Design review of the part built by this model. Coordinates are the model's own, in mm. Face numbers are marked on the shaded views. A direction names the side the tool comes from. Coordinates: 2 decimals unless noted, no trailing zeros. Loops run counter-clockwise (first coordinate to the right, second up) from the corner with the lowest first, then second, coordinate; pieces in that order, holes last. Notation, with made-up numbers: (67, -22.75) - (126, -22.75) arc R11 ccw to (126, -17.75) - close; hole circle Ø8 at (75.25, 35). An arc over 180 degrees is marked (long way). Answer in a Markdown table with one row per item. Add a question column.
(1) Clearance check with flat-ended pins moving along their axes: pin 1 (5.5 mm diameter, centred on x = 31, y = 24.5, fed in from +Z); pin 2 (1.5 mm diameter, centred on y = 5.5, z = 38, fed in from +X); pin 3 (9.5 mm diameter, centred on x = 36, y = 29, fed in from -Z). State where each tip first meets the part, or that it passes through.
(2) To check wall thickness, follow L1, parallel to Z at x = 22, y = 32; L2, parallel to Z at x = 5, y = 3. State the ranges of each line that lie inside material, in increasing order. Write a range as [from, to].
(3) We need section A-A, the plane y = 20.5. Write out the cut boundary in (x, z).
(4) We need section B-B, the plane x = 17.5. Write out the cut boundary in (y, z), plus the area to 3 significant figures.
(5) We need section C-C, the plane z = 28. Write out the cut boundary in (x, y), plus the area to 3 significant figures.
(6) We need section D-D, the plane z = 6. Write out the cut boundary in (x, y).
(7) For the marked faces 1, 2 and 3, list the 3-axis set-ups (+Z, -Z, +X, -X, +Y, -Y) from which the entire face can be reached by the end or side of a thin tool; tool diameter is ignored.
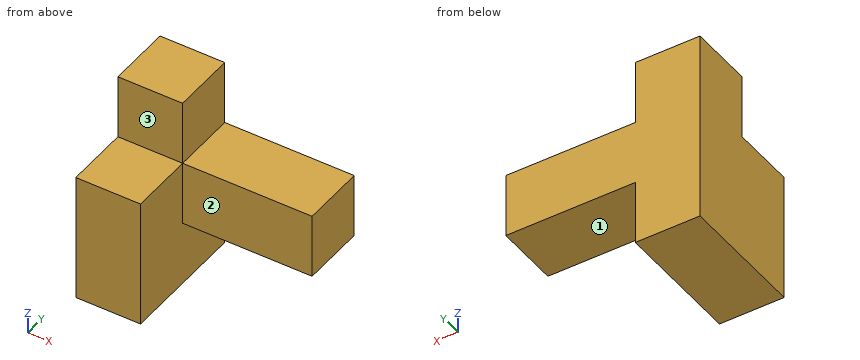
from build123d import *

# Parameters (mm, degrees)
F0_W     = 19.05
F0_H     = 38.1
F1_DEPTH = 57.15
F2_W     = 19.05
F2_H     = 19.05
F3_DEPTH = 19.05
F4_W     = 19.05
F4_H     = 19.05
F5_DEPTH = 38.1


with BuildPart() as f1:
    # F0 (on Top) → F1 (new body)
    with BuildSketch(Plane.XY):
        with Locations((9.525, 19.05)):
            Rectangle(F0_W, F0_H)
    extrude(amount=F1_DEPTH)

    # F2 (on face) → F3 (cut)
    with BuildSketch(Plane.YZ.offset(19.05)):
        with Locations((9.525, 47.625)):
            Rectangle(F2_W, F2_H)
    extrude(amount=-F3_DEPTH, mode=Mode.SUBTRACT)

    # F4 (on face) → F5 (join)
    with BuildSketch(Plane.YZ.offset(19.05)):
        with Locations((28.575, 28.575)):
            Rectangle(F4_W, F4_H)
    extrude(amount=F5_DEPTH)


solid = f1.part
Responses:
| question | item | result |
|---|---|---|
| 1 | pin 1 | stops at z = 38.1 |
| 1 | pin 2 | stops at x = 19.05 |
| 1 | pin 3 | stops at z = 19.05 |
| 2 | L1 | z = [19.05, 38.1] |
| 2 | L2 | z = [0, 38.1] |
| 3 | outline | (0, 0) - (19.05, 0) - (19.05, 19.05) - (57.15, 19.05) - (57.15, 38.1) - (19.05, 38.1) - (19.05, 57.15) - (0, 57.15) - close |
| 4 | outline | (0, 0) - (38.1, 0) - (38.1, 57.15) - (19.05, 57.15) - (19.05, 38.1) - (0, 38.1) - close |
| 4 | area | 1,810 mm2 |
| 5 | outline | (0, 0) - (19.05, 0) - (19.05, 19.05) - (57.15, 19.05) - (57.15, 38.1) - (0, 38.1) - close |
| 5 | area | 1,450 mm2 |
| 6 | outline | (0, 0) - (19.05, 0) - (19.05, 38.1) - (0, 38.1) - close |
| 7 | face 1 | -Z, +X, +Y, -Y |
| 7 | face 2 | +Z, -Z, +X, -Y |
| 7 | face 3 | +Z, +X, -X, -Y |
